Build history of the part. All positions in model axes, mm. A direction names the side the tool comes from. Round coordinates to 2 decimals unless told otherwise and drop trailing zeros. Loops run counter-clockwise (first coordinate to the right, second up) from the corner with the lowest first, then second, coordinate; pieces in that order, holes last. Notation, with made-up numbers: (85.25, 17) - (109.25, 17) arc R9 cw to (109.25, 28) - close; hole circle Ø8 at (64.5, 9.25). An arc over 180 degrees is marked (long way). Use one line per item in the form item = value. Start each with the question number.
Q1. Pin check, flat tips, straight feed: pin 1 (3 mm diameter, centred on x = 4, z = -1.5, fed in from -Y); pin 2 (4 mm diameter, centred on y = -7.5, z = 4, fed in from +X); pin 3 (5 mm diameter, centred on x = -3, y = -7, fed in from -Z). Stop position of each tip, or through.
Q2. 3-axis set-ups, long thin cutter, end or side, ignore diameter. For faces 1 (the face through (2.685, -0.428, -0.596)), 2 (the face through (-2.4, 0, 4.3)), 3 (the face through (3, -0.15, 1)), 4 (the face through (3, 0, -4)): which of +Z, -Z, +X, -X, +Y, -Y reach the whole face in a straight line?
Q3. Saw through at A-A (y = -8.5). Give the cut face in (x, z).
Q4. Drill centre lines: line 1 (X direction, y = -7.5, z = -0.75); line 2 (Y direction, x = 3.5, z = 2.25); line 3 (Z direction, x = -2.5, y = -6.25). Where is each one in solid material? Low to high.
```python
from build123d import *

# Parameters (mm, degrees)
SKETCH2_OUTSIDE_W  = 18.472
SKETCH2_OUTSIDE_H  = 18.472
CUT_EXTRUDE1_DEPTH = 19.95
CHAMFER1_SIZE      = 0.2


with BuildPart() as part:
    # Sketch1 → Revolve1 (revolve)
    with BuildSketch(Plane(origin=(0, 0, 0), x_dir=(0, 0, -1), z_dir=(1, 0, 0)), mode=Mode.PRIVATE) as revolve1_sk:
        with BuildLine():
            Line((0, 4), (4.5, 4))
            Line((4.5, 4), (5.675, 3.572334975))
            Line((5.675, 3.572334975), (5.675, 0))
            Line((5.675, 0), (4.75, 0))
            Line((4.75, 0), (4.4, -0.15))
            Line((4.4, -0.15), (3, -0.15))
            ThreePointArc((3, -0.15), (2.93268544, -0.1629636), (2.875, -0.2))
            Line((2.875, -0.2), (2.75, -0.2))
            Line((2.75, -0.2), (2.75, -0.65))
            Line((2.75, -0.65), (3, -0.9))
            Line((3, -0.9), (3, -15.45))
            Line((3, -15.45), (2.5, -15.95))
            Line((2.5, -15.95), (0, -15.95))
            Line((0, -15.95), (0, 4))
        make_face()
    revolve(revolve1_sk.sketch.rotate(Axis((0, 15.969730791, 0), (0, -1, 0)), 180), axis=Axis((0, 15.969730791, 0), (0, -1, 0)))

    # Sketch2 outside → Cut-Extrude1 (cut)
    with BuildSketch(Plane(origin=(0, 4, 0), x_dir=(1, 0, 0), z_dir=(0, 1, 0))):
        Rectangle(SKETCH2_OUTSIDE_W, SKETCH2_OUTSIDE_H)
        Polygon((2.857883832, -4.95), (5.715767665, 0), (2.857883832, 4.95), (-2.857883832, 4.95), (-5.715767665, 0), (-2.857883832, -4.95), align=None, mode=Mode.SUBTRACT)
    extrude(amount=-CUT_EXTRUDE1_DEPTH, mode=Mode.SUBTRACT)

    # Chamfer1
    # the kernel refuses this chamfer: 0.2 mm, written as the material it takes off along each edge
    with BuildSketch(Plane(origin=(-2.641932243, 0, 5.324039125), x_dir=(-0.023812127644090332, 0.9996219169112968, 0.01374793830529327), z_dir=(-0.4999999999999996, 0, -0.8660254037844389)), Plane(origin=(3.289787011, 0, 4.95), x_dir=(0, 0.9996219169112966, 0.027495876610587326), z_dir=(-1, 0, 0)), Plane(origin=(5.931719254, 0, -0.374039125), x_dir=(0.023812127644088587, 0.9996219169112968, 0.013747938305292286), z_dir=(-0.5000000000000003, 0, 0.8660254037844386)), Plane(origin=(-5.931719254, 0, 0.374039125), x_dir=(-0.023812127644091206, 0.9996219169112966, -0.013747938305293793), z_dir=(0.5000000000000002, 0, -0.8660254037844386)), Plane(origin=(-3.289787011, 0, -4.95), x_dir=(0, 0.9996219169112966, -0.027495876610587326), z_dir=(1, 0, 0)), Plane(origin=(2.641932243, 0, -5.324039125), x_dir=(0.02381212764409033, 0.9996219169112968, -0.013747938305293275), z_dir=(0.49999999999999994, 0, 0.8660254037844388))) as chamfer1_piece_1:
        Polygon((CHAMFER1_SIZE * 0.999621916911, CHAMFER1_SIZE * 0.0274958766106), (-CHAMFER1_SIZE * 0.0274958766106, CHAMFER1_SIZE * 0.999621916911), (0, 0), align=None)
    extrude(amount=6.579574023, mode=Mode.SUBTRACT)


solid = part.part
```
Report:
q1.pin_1 = -15.68
q1.pin_2 = 2.24
q1.pin_3 = -2.96
q2.face_1 = none
q2.face_2 = +Z, -X, -Y
q2.face_3 = -Y
q2.face_4 = -Z, +X, -Y
q3.outline = circle Ø6 at (0, 0)
q4.line_1 = -2.9 to 2.9
q4.line_2 = -0.15 to 4
q4.line_3 = -1.66 to 1.66
